Geometry: see drawing. Coordinates: mm, zero at the bounding-box minimum. Give positions to 0.01 mm unless a question says otherwise; leave off trailing zeros. Loops run counter-clockwise (first coordinate to the right, second up) from the corner with the lowest first, then second, coordinate; pieces in that order, holes last. Notation, with made-up numbers: M 13,-24 L 44,-24 A18 ccw 44,5 Z; hole C -38.5,56 d9. An arc over 180 degrees is marked long. Use a Markdown table: item, result. Add a question column.
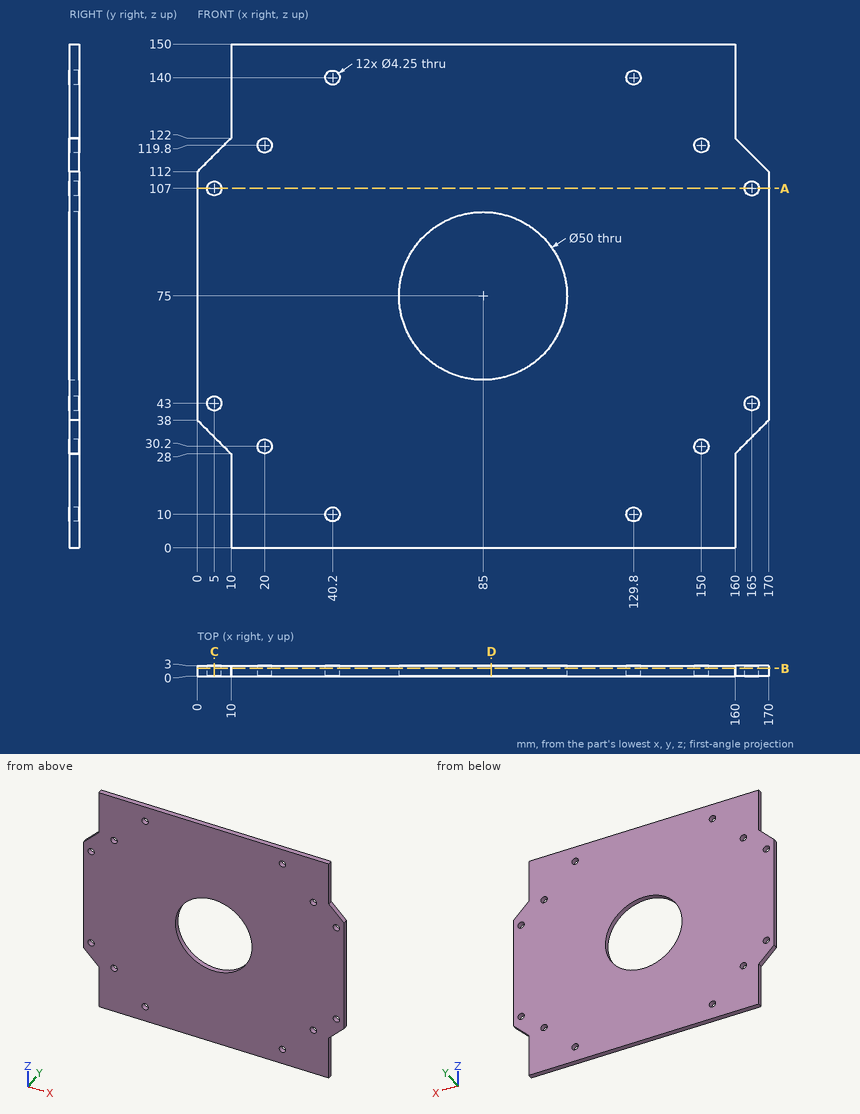
1) Section query D-D, the plane x = 87.5. Return the cut outline in (y, z).
2) Ray query, line 1 (X direction, y = 0.65, z = 10) (3 decimals); line 2 (Z direction, x = 129.8, y = 2.2) (3 decimals); line 3 (X direction, y = 0.9, z = 107) (3 decimals). Return the intervals inside material, ascending. Write a range as [from, to].
3) Contact query for flat-ended pins moving along their axis: P1, Ø5, axis at x = 65, z = 132, coming from the -Y side; P2, Ø3.5, axis at x = 165, z = 43, coming from the +Y side; P3, Ø0.9, axis at y = 1.5, z = 137, coming from the -X side. Output: stop coordinate, or through.
4) Section query A-A, the plane z = 107. Return the cut outline in (x, y) (3 decimals).
5) Section query B-B, the plane y = 2.3. State how many separate pieces and enclosed holes the cut face has, and give its area (3 significant figures).
6) Section query C-C, the plane x = 5. Return the cut outline in (y, z) (3 decimals), and give its area (4 significant figures).
Entries:
| question | item | result |
|---|---|---|
| 1 | outline | M 0,0 L 3,0 L 3,50.13 L 0,50.13 Z; M 0,99.87 L 3,99.87 L 3,150 L 0,150 Z |
| 2 | line 1 | x = [10, 38.075], [42.325, 127.675], [131.925, 160] |
| 2 | line 2 | z = [0, 7.875], [12.125, 137.875], [142.125, 150] |
| 2 | line 3 | x = [0, 2.875], [7.125, 162.875], [167.125, 170] |
| 3 | P1 | stops at y = 0 |
| 3 | P2 | passes through |
| 3 | P3 | stops at x = 10 |
| 4 | outline | M 0,0 L 2.875,0 L 2.875,3 L 0,3 Z; M 7.125,0 L 162.875,0 L 162.875,3 L 7.125,3 Z; M 167.125,0 L 170,0 L 170,3 L 167.125,3 Z |
| 5 | separate pieces | 1 |
| 5 | enclosed holes | 13 |
| 5 | area | 22,000 mm² |
| 6 | outline | M 0,33 L 3,33 L 3,40.875 L 0,40.875 Z; M 0,45.125 L 3,45.125 L 3,104.875 L 0,104.875 Z; M 0,109.125 L 3,109.125 L 3,117 L 0,117 Z |
| 6 | area | 226.5 mm² |
